Geometry: final body of the model. Coordinates: model frame, mm. Face numbers are marked on the shaded views. A direction names the side the tool comes from. Give positions to 0.01 mm unless a question says otherwise; leave off trailing zeros. Write each loop counter-clockwise with the first axis right and the second up, starting at its lowest first coordinate (ties: lowest second). Pieces come first, ordered by that corner, then holes. Notation, with made-up numbers: M 61,23.5 L 111,23.5 A20 ccw 111,41.5 Z; hole C 37.5,3 d10. An arc over 180 degrees is marked long. Use a Markdown table: item, result. Add a question column.
(1) Cut plane B-B (x = 4.5). Output: boundary loops of the cut face in (y, z).
(2) Cut plane C-C (z = -2.25). Output: boundary loops of the cut face in (x, y).
(3) Material intervals for L1, parallel to X at y = 0.1, z = -7; L2, parallel to Z at x = 4.75, y = 0.1; L3, parallel to X at y = 0.15, z = -6.25, sorted ascending.
(4) Reachability of the marked faces 1 and 2 from +Z, -Z, +X, -X, +Y, -Y: full face, straight path, thin tool, end or side. Return the list, or none.
(5) Cut plane A-A (z = -7). Output: boundary loops of the cut face in (x, y), plus the area to 4 significant figures.
(6) Draft query along X for the marked faces 3 and 4. Return one class per face: released by +X, released by -X, zero draft, split by the parting line, or undercut.
(7) Cut plane D-D (x = 5.75). Output: boundary loops of the cut face in (y, z), plus the area to 3 significant figures.
```python
from build123d import *

# Parameters (mm, degrees)
SKETCH1_W           = 0.6
SKETCH1_H           = 1.7
BOSS_EXTRUDE1_DEPTH = 0.4
FILLET2_R           = 1
SKETCH2_W           = 1.5
SKETCH2_H           = 8.5
CUT_EXTRUDE1_DEPTH  = 0.05


with BuildPart() as part:
    # Sketch1 → Boss-Extrude1 (new body)
    with BuildSketch(Plane(origin=(0, 0, 0), x_dir=(1, 0, 0), z_dir=(0, 1, 0))):
        Polygon((0, 0), (7, 0), (7, 8.5), (0.3, 8.5), (0.3, 6.5), (0, 6.5), (0, 4.5), (0.3, 4.5), (0.3, 1.5), (0, 1.5), align=None)
        with Locations((4.7, 6.65)):
            Rectangle(SKETCH1_W, SKETCH1_H, mode=Mode.SUBTRACT)
        with Locations((6.2, 3.25)):
            Rectangle(SKETCH1_W, SKETCH1_H, mode=Mode.SUBTRACT)
    extrude(amount=BOSS_EXTRUDE1_DEPTH)

    # Fillet2
    fillet2_edges = [part.edges().sort_by_distance(p)[0] for p in [
        (0.3, 0.2, -8.5),
        (7, 0.2, -8.5),
        (7, 0.2, 0),
    ]]
    fillet(fillet2_edges, radius=FILLET2_R)

    # Sketch2 → Cut-Extrude1 (cut)
    with BuildSketch(Plane.XZ):
        with BuildLine():
            Line((6.448166538, -2.4), (6.448166538, -5.1))
            ThreePointArc((6.448166538, -5.1), (6.314670512, -5.458517669), (5.979203511, -5.642414377))
            Line((5.979203511, -5.642414377), (4.9, -5.8))
            Line((4.9, -5.8), (4.9, -8.5))
            ThreePointArc((4.9, -8.5), (4.4, -9), (3.9, -8.5))
            Line((3.9, -8.5), (3.9, -5.8))
            Line((3.9, -5.8), (3.9, -5.367707784))
            ThreePointArc((3.9, -5.367707784), (4.021765938, -5.040692502), (4.327755978, -4.872954511))
            Line((4.327755978, -4.872954511), (5.448166538, -4.709351823))
            Line((5.448166538, -4.709351823), (5.448166538, -2.4))
            Line((5.448166538, -2.4), (5.448166538, 0))
            Line((5.448166538, 0), (6.448166538, 0))
            Line((6.448166538, 0), (6.448166538, -2.4))
        make_face()
        with Locations((0.75, -4.25)):
            Rectangle(SKETCH2_W, SKETCH2_H)
    extrude(amount=-CUT_EXTRUDE1_DEPTH, mode=Mode.SUBTRACT)


solid = part.part
```
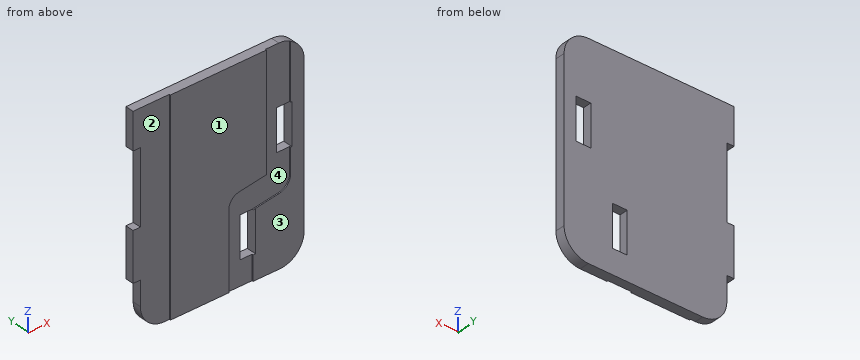
Answer list:
| question | item | result |
|---|---|---|
| 1 | outline | M 0,-4.85 L 0.05,-4.85 L 0.05,-5.8 L 0.4,-5.8 L 0.4,0 L 0,0 Z; M 0.05,-8.5 L 0.4,-8.5 L 0.4,-7.5 L 0.05,-7.5 Z |
| 2 | outline | M 0.3,0.05 L 1.5,0.05 L 1.5,0 L 5.45,0 L 5.45,0.05 L 6.45,0.05 L 6.45,0 L 7,0 L 7,0.4 L 0.3,0.4 Z |
| 3 | L1 | 0.3 to 4.4, 5 to 7 |
| 3 | L2 | -8.5 to -7.5, -5.8 to 0 |
| 3 | L3 | 0 to 4.4, 5 to 7 |
| 4 | face 1 | +Z, -Z, +X, -X, -Y |
| 4 | face 2 | +Z, -Z, -X, -Y |
| 5 | outline | M 0.3,0.05 L 1.5,0.05 L 1.5,0 L 3.9,0 L 3.9,0.05 L 4.4,0.05 L 4.4,0.4 L 0.3,0.4 Z; M 5,0 L 7,0 L 7,0.4 L 5,0.4 Z |
| 5 | area | 2.355 mm² |
| 6 | face 3 | zero draft |
| 6 | face 4 | undercut |
| 7 | outline | M 0,-8.5 L 0.4,-8.5 L 0.4,0 L 0.05,0 L 0.05,-5.68 L 0,-5.68 Z |
| 7 | area | 3.12 mm² |
